Part model, mm, in its own coordinate system. Round coordinates to 2 decimals unless told otherwise and drop trailing zeros. Loops run counter-clockwise (first coordinate to the right, second up) from the corner with the lowest first, then second, coordinate; pieces in that order, holes last.
(1) Flat gauge pins, fed straight in: pin 1 (2 mm diameter, centred on y = 13.5, z = 2, fed in from -X); pin 2 (1.8 mm diameter, centred on x = 0, y = 6, fed in from -Z); pin 3 (1.5 mm diameter, centred on x = -1, y = 20, fed in from +Z). Where does each tip first touch, or does it go through?
(2) Cut at C-C on y = 27. List the corners of the cut face in (x, z).
(3) Cut at B-B on z = -1.1. List the corners of the cut face in (x, y) (3 decimals), then the cut area to 3 significant figures.
(4) Cut at D-D on z = 0.75. List the corners of the cut face in (x, y).
(5) Cut at A-A on x = 0. List the corners of the cut face in (y, z).
(6) Mould opens along Y. For faces 1 (the face through (-1.43, 6.45, 0.28)), 2 (the face through (0, 2, -2)), 3 (the face through (0, 0, 0)), 4 (the face through (0, 42.7, 0)) say: +Y half, -Y half, draft (parallel to the pull), parting line (faces both ways), or undercut.
(7) Probe probe 1 along Y at (x, z) = (0, 1); probe 2 along Y at (x, z) = (-0.55, -0.85); probe 3 along X at (y, z) = (5.5, 1.9). List the from-to ranges inside material, lowest first.
from build123d import *

# Parameters (mm, degrees)
BOSS_EXTRUDE1_DEPTH     = 42.7
CUT_EXTRUDE1_DEPTH      = 44.009185066
CUT_EXTRUDE1_DEPTH_BACK = 44.009185066
SKETCH2_R               = 1.5


with BuildPart() as part:
    # Sketch1 → Boss-Extrude1 (new body)
    with BuildSketch(Plane(origin=(0, 0, 0), x_dir=(1, 0, 0), z_dir=(0, 1, 0))):
        with BuildLine():
            Line((1.5, 2), (-1.5, 2))
            ThreePointArc((-1.5, 2), (-1.118033989, -2.236067977), (2.5, 0))
            ThreePointArc((2.5, 0), (2.236067977, 1.118033989), (1.5, 2))
        make_face()
    extrude(amount=BOSS_EXTRUDE1_DEPTH)

    # Sketch2 → Cut-Extrude1 (cut, two sides: drawn at the far end of the back side and taken through both)
    with BuildSketch(Plane(origin=(0, 0, -2), x_dir=(-1, 0, 0), z_dir=(0, 0, -1)).offset(-CUT_EXTRUDE1_DEPTH_BACK)):
        with Locations((0, 6)):
            Circle(SKETCH2_R)
    extrude(amount=CUT_EXTRUDE1_DEPTH + CUT_EXTRUDE1_DEPTH_BACK, mode=Mode.SUBTRACT)


solid = part.part
Final values:
1. pin 1: stops at x = -2.29
1. pin 2: passes through
1. pin 3: stops at z = 2.49
2. outline: (-1.5, -2) - (1.5, -2) arc R2.5 ccw (long way) to start
3. outline: (-2.245, 0) - (2.245, 0) - (2.245, 42.7) - (-2.245, 42.7) - close; hole circle Ø3 at (0, 6)
3. area: 185 mm2
4. outline: (-2.38, 0) - (2.38, 0) - (2.38, 42.7) - (-2.38, 42.7) - close; hole circle Ø3 at (0, 6)
5. outline: (0, -2) - (4.5, -2) - (4.5, 2.5) - (0, 2.5) - close; (7.5, -2) - (42.7, -2) - (42.7, 2.5) - (7.5, 2.5) - close
6. face 1: undercut
6. face 2: draft
6. face 3: -Y half
6. face 4: +Y half
7. probe 1: y = 0 to 4.5, 7.5 to 42.7
7. probe 2: y = 0 to 4.6, 7.4 to 42.7
7. probe 3: x = -1.62 to -1.41, 1.41 to 1.62
